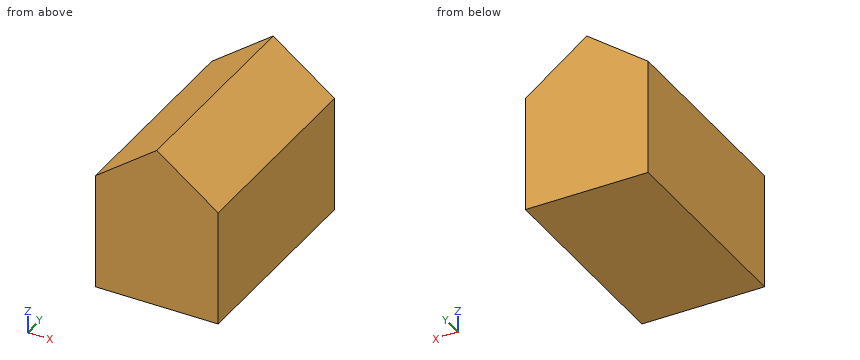
```python
from build123d import *

# Parameters (mm, degrees)
F0_W     = 89.191474
F0_H     = 84.23639
F1_DEPTH = 76.2


with BuildPart() as f1:
    # F0 (on Front) → F1 (new body, symmetric)
    with BuildSketch(Plane.XZ):
        Polygon((0, 75.346395), (-44.595737, 42.118195), (44.595737, 42.118195), align=None)
        Rectangle(F0_W, F0_H)
    extrude(amount=F1_DEPTH, both=True)


solid = f1.part
```
Check sheet for the modelled part. Datum: model origin and axes. Units: mm. Give positions to 0.01 mm unless a question says otherwise; leave off trailing zeros. Write each loop counter-clockwise with the first axis right and the second up, starting at its lowest first coordinate (ties: lowest second). Pieces come first, ordered by that corner, then holes.
Item 1: Cross-section at C-C (x = 15.5). Enter the section's corners in (y, z).
Item 2: Gauge pin test, flat ends, axial feed: pin 1 (2 mm diameter, centred on x = -15, y = -24.5, fed in from +Z) (3 decimals); pin 2 (5 mm diameter, centred on y = -50, z = 55, fed in from -X); pin 3 (2 mm diameter, centred on x = 5, y = 13.5, fed in from +Z). Record the tip position at first contact, or that the pin passes through.
Item 3: Cross-section at A-A (y = -8.5). Enter the section's corners in (x, z).
Item 4: Scan lines: L1, parallel to Z at x = -24, y = 58; L2, parallel to X at y = -62.5, z = 64.5; L3, parallel to Z at x = -29, y = 42. Record each from-to range of solid material in increasing order.
Item 5: Cross-section at B-B (z = 59.5). Enter the section's corners in (x, y), and give its area (3 significant figures).
Report:
1. outline: (-76.2, -42.12) - (76.2, -42.12) - (76.2, 63.8) - (-76.2, 63.8) - close
2. pin 1: stops at z = 64.915
2. pin 2: stops at x = -30.66
2. pin 3: stops at z = 72.37
3. outline: (-44.6, -42.12) - (44.6, -42.12) - (44.6, 42.12) - (0, 75.35) - (-44.6, 42.12) - close
4. L1: z = -42.12 to 57.46
4. L2: x = -14.56 to 14.56
4. L3: z = -42.12 to 53.74
5. outline: (-21.27, -76.2) - (21.27, -76.2) - (21.27, 76.2) - (-21.27, 76.2) - close
5. area: 6,480 mm2
